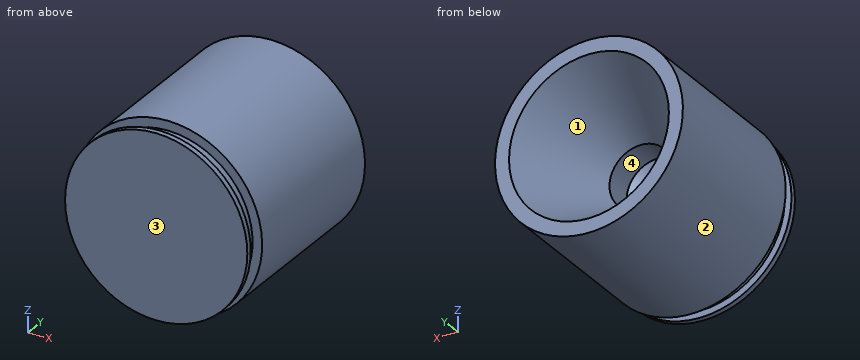
from build123d import *


with BuildPart() as f2:
    # F1 (on face) → F2 (revolve)
    with BuildSketch(Plane.YZ):
        Polygon((0, 35), (0, 0), (20.204075, 0), (26.879636, 11.11), (36.879636, 11.11), (67, 28.5), (67, 35), align=None)
    revolve(axis=Axis((0, 35.295283, 0), (0, 1, 0)))

    # F3 (on Right) → F4 (revolve, cut)
    with BuildSketch(Plane.YZ):
        Polygon((7, 33.5), (68.52591, 33.5), (69.647816, 44.953279), (0, 44.953279), (0, 32.5), (2, 32.5), (2, 30.1), (7, 30.1), align=None)
    revolve(axis=Axis((0, 56.397552, 0), (0, 1, 0)), mode=Mode.SUBTRACT)


solid = f2.part
Work out the finished part from the listing and answer in its coordinate system (mm). Face numbers are marked on the shaded views. Coordinates: 2 decimals unless noted, no trailing zeros. Write each loop counter-clockwise with the first axis right and the second up, starting at its lowest first coordinate (ties: lowest second). Pieces come first, ordered by that corner, then holes. Notation, with made-up numbers: M 37.5,76 L 49.5,76 A30 cw 49.5,113 Z; hole C 5.5,50.5 d5. An arc over 180 degrees is marked long. Use one line per item in the form item = value. Start each with the question number.
1. The part is cut by section B-B (y = 49). Give the vertices of the cut face in (x, z).
2. Straight lines are drawn through the part: probe 1 along X at (y, z) = (31.75, 0); probe 2 along Y at (x, z) = (24, 20); probe 3 along X at (y, z) = (53, -7.5). For each, find the intervals that lie inside material, in ascending order. Write a range as from..to.
3. Each of these flat-tipped pins is pushed along its axis until it touches: P1, Ø3, axis at y = 21, z = -8.5, coming from the -X side; P2, Ø5, axis at x = -22.5, z = 9.5, coming from the +Y side; P3, Ø5, axis at x = -17, z = -16.5, coming from the +Y side. Where does it stop, or does it pass through?
4. The mould has two halves that part along Z. Classify the marked faces 1, 2, 3 and 4: released by +Z, released by -Z, zero draft, split by the parting line, or undercut.
5. The part is cut by section A-A (y = 19). Give the vertices of the cut face in (x, z).
Evaluation:
q1.outline = C 0,0 d67; hole C 0,0 d36.22
q2.probe_1 = -33.5..-11.11, 11.11..33.5
q2.probe_2 = 0..2, 7..67
q2.probe_3 = -32.65..-18.99, 18.99..32.65
q3.P1 = -32.76
q3.P2 = 64.27
q3.P3 = 63
q4.face_1 = undercut
q4.face_2 = split by the parting line
q4.face_3 = zero draft
q4.face_4 = undercut
q5.outline = C 0,0 d67
